CAD build for the part. Positions are in the model's coordinates, mm. A direction names the side the tool comes from. Give positions to 0.01 mm unless a question says otherwise; leave off trailing zeros. Loops run counter-clockwise (first coordinate to the right, second up) from the corner with the lowest first, then second, coordinate; pieces in that order, holes last. Notation, with made-up numbers: M -12,-22 L 6,-22 A12 cw 6,-11 Z; hole C 31,17 d9. An arc over 180 degrees is marked long. Answer as CSV lines item,"result".
from build123d import *

# Parameters (mm, degrees)
F0_W     = 203.2
F0_H     = 101.6
F1_DEPTH = 101.6
F2_W     = 50.8
F2_H     = 50.8
F3_DEPTH = 76.2
F5_DEPTH = 50.8
F6_R     = 25.4
F7_R     = 12.7
F8_DEPTH = 38.1


with BuildPart() as f1:
    # F0 (on Front) → F1 (new body)
    with BuildSketch(Plane.XZ):
        with Locations((101.6, 50.8)):
            Rectangle(F0_W, F0_H)
    extrude(amount=F1_DEPTH)

    # F2 (on face) → F3 (cut)
    with BuildSketch(Plane.XZ.offset(101.6)):
        with Locations((25.4, 25.4)):
            Rectangle(F2_W, F2_H)
        with Locations((177.8, 25.4)):
            Rectangle(F2_W, F2_H)
    extrude(amount=-F3_DEPTH, mode=Mode.SUBTRACT)

    # F4 (on face) → F5 (cut)
    with BuildSketch(Plane.XZ.offset(101.6)):
        Polygon((0, 50.8), (50.8, 50.8), (152.4, 50.8), (203.2, 50.8), (203.2, 101.6), (0, 101.6), align=None)
    extrude(amount=-F5_DEPTH, mode=Mode.SUBTRACT)

    # F6
    f6_edges = [f1.edges().sort_by_distance(p)[0] for p in [
        (203.2, -25.4, 101.6),
        (0, -25.4, 101.6),
    ]]
    fillet(f6_edges, radius=F6_R)

    # F7 (on face) → F8 (cut)
    with BuildSketch(Plane.XZ.offset(50.8)):
        with Locations((25.4, 76.2)):
            Circle(F7_R)
        with Locations((177.8, 76.2)):
            Circle(F7_R)
    extrude(amount=-F8_DEPTH, mode=Mode.SUBTRACT)


solid = f1.part
1) Drill centre lines: line 1 (X direction, y = -26, z = 76); line 2 (X direction, y = -20, z = 81); line 3 (X direction, y = -97, z = 7). Where is each one in solid material? Low to high. Write a range as from..to.
Answer below:
line 1,"x = 0..12.7, 38.1..165.1, 190.5..203.2"
line 2,"x = 0.46..13.64, 37.16..166.04, 189.56..202.74"
line 3,"x = 50.8..152.4"
2) Band-saw the part on B-B on z = 47. Give the cut face in (x, y).
Answer below:
outline,"M 0,-25.4 L 50.8,-25.4 L 50.8,-101.6 L 152.4,-101.6 L 152.4,-25.4 L 203.2,-25.4 L 203.2,0 L 0,0 Z"
3) Band-saw the part on C-C on x = 96. Give the cut face in (y, z).
Answer below:
outline,"M -101.6,0 L 0,0 L 0,101.6 L -50.8,101.6 L -50.8,50.8 L -101.6,50.8 Z"
4) Flat gauge pins, fed straight in: pin 1 (15 mm diameter, centred on x = 25.4, z = 76.2, fed in from -Y); pin 2 (1.5 mm diameter, centred on x = 84, z = 76.5, fed in from -Y); pin 3 (7.5 mm diameter, centred on x = 31, y = -34, fed in from -Z). Where does each tip first touch, or does it go through?
Answer below:
pin 1,"stops at y = -12.7"
pin 2,"stops at y = -50.8"
pin 3,"stops at z = 50.8"
5) Which spindle directions (+Z, -Z, +X, -X, +Y, -Y) get a long thin tool onto all of the face, cutting with end or side? Do faces 1 (the face through (177, -38, 50.8)), 2 (the face through (100, 0, 52)), 3 (the face through (100, -50.8, 77)), 4 (the face through (25, -25.4, 26)), 5 (the face through (25, -12.7, 76)). Say none if no direction does.
Answer below:
face 1,"-Z, +X, -Y"
face 2,"+Z, -Z, +X, -X, +Y"
face 3,"+Z, +X, -X, -Y"
face 4,"-Z, -X, -Y"
face 5,"-Y"
6) Band-saw the part on D-D on y = -55. Give the cut face in (x, z), and give its area (3 significant figures).
Answer below:
outline,"M 50.8,0 L 152.4,0 L 152.4,50.8 L 50.8,50.8 Z"
area,"5,160 mm^2"
7) Mould opens along X. For faces 6 (the face through (152.4, -64, 25)), 7 (the face through (22.65, -32.02, 63.8)), 8 (the face through (101, -77, 50.8)) say: +X half, -X half, draft (parallel to the pull), parting line (faces both ways), or undercut.
Answer below:
face 6,"+X half"
face 7,"undercut"
face 8,"draft"
8) Band-saw the part on A-A on y = -33. Give the cut face in (x, z), and give its area (3 significant figures).
Answer below:
outline,"M 0,50.8 L 50.8,50.8 L 50.8,0 L 152.4,0 L 152.4,50.8 L 203.2,50.8 L 203.2,76.2 A25.4 ccw 177.8,101.6 L 25.4,101.6 A25.4 ccw 0,76.2 Z; hole C 25.4,76.2 d25.4; hole C 177.8,76.2 d25.4"
area,"14,200 mm^2"
